```python
from build123d import *

# Parameters (mm, degrees)
BOSS_EXTRUDE1_DEPTH   = 3.175
F_8_CLEARANCE_HOLE1_D = 4.3053


with BuildPart() as part:
    # Sketch1 → Boss-Extrude1 (new body)
    with BuildSketch(Plane(origin=(0, 0, 0), x_dir=(1, 0, 0), z_dir=(0, 1, 0))):
        Polygon((126.25, 0), (0, 0), (0, 126.25), (31.75, 126.25), (126.25, 31.75), align=None)
    extrude(amount=BOSS_EXTRUDE1_DEPTH)

    # #8 Clearance Hole1 (through all)
    with Locations(Plane(origin=(0, 3.175, 0), x_dir=(1, 0, 0), z_dir=(0, 1, 0))):
        with Locations((15.875, 61.75), (15.875, 80.75), (6.375, 90.25), (25.375, 90.25), (15.875, 99.75), (15.875, 118.75), (118.75, 15.875), (99.75, 15.875), (90.25, 25.375), (90.25, 6.375), (80.75, 15.875), (61.75, 15.875)):
            Hole(F_8_CLEARANCE_HOLE1_D / 2)


solid = part.part
```
CAD build for the part. Positions are in the model's coordinates, mm. Round coordinates to 2 decimals unless told otherwise and drop trailing zeros. Order: outer loops, then holes, each group sorted by start corner. A loop starts at its lowest first (then second) coordinate and runs counter-clockwise, first axis right, second up. Notation, with made-up numbers: (70.25, 33) -> (115.25, 33) arc R14 cw to (115.25, 49) -> close; hole circle Ø10 at (50.5, -4.5). An arc over 180 degrees is marked (long way). One line per question, with ' | ' between items.
Q1. Slice it at A-A (z = -61.75). Write the cut outline in (x, y) (3 decimals), then the cut area to 3 significant figures.
Completed:
outline: (0, 0) -> (13.722, 0) -> (13.722, 3.175) -> (0, 3.175) -> close; (18.028, 0) -> (96.25, 0) -> (96.25, 3.175) -> (18.028, 3.175) -> close | area: 292 mm^2
Q2. Probe probe 1 along Z at (x, y) = (17.5, 1.25); probe 2 along X at (y, z) = (2.4, -80.75); probe 3 along Z at (x, y) = (61, 2.4). List the from-to ranges inside material, lowest first.
Completed:
probe 1: z = -126.25 to -120.16, -117.34 to -101.16, -98.34 to -82.16, -79.34 to -63.16, -60.34 to 0 | probe 2: x = 0 to 13.72, 18.03 to 77.25 | probe 3: z = -97 to -17.89, -13.86 to 0
Q3. Slice it at D-D (y = 2.3). Give the number of separate pieces and of enclosed holes in the cut face, then the cut area to 3 significant figures.
Completed:
separate pieces: 1 | enclosed holes: 12 | area: 11,300 mm^2
Q4. Drop flat-ended pins along their axis: pin 1 (1.5 mm diameter, centred on y = 2.5, z = -34.5, fed in from +X); pin 2 (1.5 mm diameter, centred on x = 40, y = 1, fed in from -Z). Give the stop position or say it passes through.
Completed:
pin 1: stops at x = 124.25 | pin 2: stops at z = -118.75
Q5. Two-plate mould, pull along X, no slides. Class faces 1 (the cylindrical face through (59.697, 1.565, -16.522)), 2 (the flat face through (0, 2, -62)), 3 (the cylindrical face through (16.34, 1.57, -78.65)), 4 (the flat face through (16, 2, -126.25)): released by +X, released by -X, zero draft, split by the parting line, or undercut.
Completed:
face 1: undercut | face 2: released by -X | face 3: undercut | face 4: zero draft
Q6. Slice it at B-B (z = -90.25). Write the cut outline in (x, y) (3 decimals), then the cut area to 3 significant figures.
Completed:
outline: (0, 0) -> (4.222, 0) -> (4.222, 3.175) -> (0, 3.175) -> close; (8.528, 0) -> (23.222, 0) -> (23.222, 3.175) -> (8.528, 3.175) -> close; (27.528, 0) -> (67.75, 0) -> (67.75, 3.175) -> (27.528, 3.175) -> close | area: 188 mm^2
Q7. Slice it at C-C (x = 118.75). Write the cut outline in (y, z) (3 decimals), then the cut area to 3 significant figures.
Completed:
outline: (0, -39.25) -> (3.175, -39.25) -> (3.175, -18.028) -> (0, -18.028) -> close; (0, -13.722) -> (3.175, -13.722) -> (3.175, 0) -> (0, 0) -> close | area: 111 mm^2
